Can you work these out from the model? Positions are in its coordinate system, mm. Round coordinates to 2 decimals unless told otherwise and drop trailing zeros. Write each loop counter-clockwise with the first axis right and the second up, starting at its lowest first coordinate (ties: lowest second). Pieces come first, ordered by that corner, then holes. Notation, with made-up numbers: M 74,-15 L 90,-15 A23 cw 90,12 Z; hole C 69,16 d11. An arc over 180 degrees is marked long. Answer in a Markdown table with one row per item. Add a question column.
(1) I'm going to push flat-ended pins straight in: pin 1 (4.5 mm diameter, centred on y = 8, z = -20, fed in from -X); pin 2 (7.5 mm diameter, centred on y = 10, z = -154.5, fed in from +X); pin 3 (4.5 mm diameter, centred on x = 4.5, z = -270.5, fed in from +Y). Where does each tip first touch, or does it pass through?
(2) If I drill on probe 1 along Z at (x, y) = (-0.65, 8); probe 2 along Y at (x, z) = (-1.4, -414); probe 3 along Y at (x, z) = (6, -258), over which ranges is the centre line in solid material (lowest first)?
(3) Suppose I cut it at A-A, the plane z = -174. Write out the boundary of the cut face in (x, y).
(4) Suppose I cut it at B-B, the plane x = 3.5. Write out the boundary of the cut face in (y, z), then the cut area to 3 significant figures.
from build123d import *

# Parameters (mm, degrees)
EXTRUDE_1_DEPTH     = 434
SKETCH_2_R          = 2.5
CUT_EXTRUDE_1_DEPTH = 435.453679925
SKETCH_3_W          = 2
SKETCH_3_H          = 2
EXTRUDE_2_DEPTH     = 434


with BuildPart() as part:
    # Эскиз1 → Бобышка-Вытянуть1 (new body)
    with BuildSketch(Plane.XY):
        Polygon((0, 0), (0, 13), (-2, 13), (-2, -2), (13, -2), (13, 0), align=None)
    extrude(amount=-EXTRUDE_1_DEPTH)

    # Эскиз2 → Вырез-Вытянуть1 (cut, through all)
    with BuildSketch(Plane.ZY.offset(2)):
        with Locations(Location((-20, 8, 0), (0, 0, 270))):
            Circle(SKETCH_2_R)
        with Locations(Location((-414, 8, 0), (0, 0, 270))):
            Circle(SKETCH_2_R)
    extrude(amount=-CUT_EXTRUDE_1_DEPTH, mode=Mode.SUBTRACT)

    # Эскиз3 → Бобышка-Вытянуть2 (add)
    with BuildSketch(Plane(origin=(0, 0, -434), x_dir=(-1, 0, 0), z_dir=(0, 0, -1))):
        with Locations((1, 14)):
            Rectangle(SKETCH_3_W, SKETCH_3_H)
        with Locations((-14, -1)):
            Rectangle(SKETCH_3_W, SKETCH_3_H)
    extrude(amount=-EXTRUDE_2_DEPTH)


solid = part.part
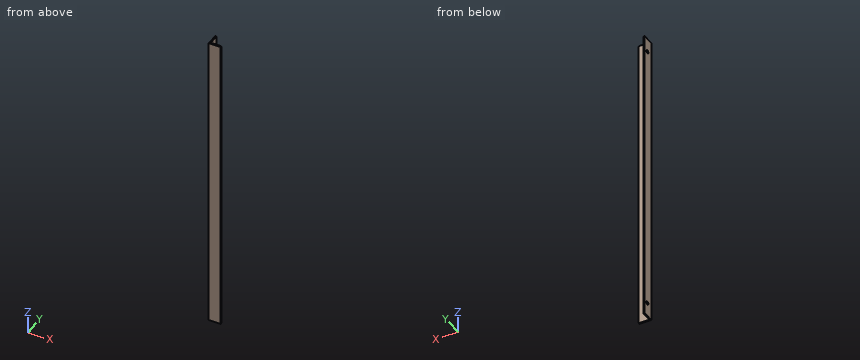
Calculated:
| question | item | result |
|---|---|---|
| 1 | pin 1 | through |
| 1 | pin 2 | x = 0 |
| 1 | pin 3 | y = 0 |
| 2 | probe 1 | -434 to -416.5, -411.5 to -22.5, -17.5 to 0 |
| 2 | probe 2 | -2 to 5.5, 10.5 to 15 |
| 2 | probe 3 | -2 to 0 |
| 3 | outline | M -2,-2 L 15,-2 L 15,0 L 0,0 L 0,15 L -2,15 Z |
| 4 | outline | M -2,-434 L 0,-434 L 0,0 L -2,0 Z |
| 4 | area | 868 mm² |
